Here's how the part is built. I have some questions about the finished solid (model axes, mm). Coordinates: 2 decimals unless noted, no trailing zeros. Write each loop counter-clockwise with the first axis right and the second up, starting at its lowest first coordinate (ties: lowest second). Pieces come first, ordered by that corner, then holes.
Item 1: We'd pull the mould along Z, two halves only. Please class faces 1 (the face through (0, 1, 400)), 2 (the face through (-0.705, 3.479, 88.173)), 3 (the face through (1.4, 1.958, 61.4)), 4 (the face through (0, 4.958, 197)): +Z half, -Z half, draft (parallel to the pull), parting line (faces both ways), or undercut.
Item 2: I'm going to push flat-ended pins straight in: pin 1 Ø1 at (x, z) = (-2.5, 260.5) entering from +Y; pin 2 Ø3 at (y, z) = (2.5, 318.5) entering from -X; pin 3 Ø3 at (x, z) = (0, 135) entering from +Y. Where does each tip first touch, or does it pass through?
Item 3: If we section it at A-A (y = 3.5): Count the separate pieces of the cut face and the enclosed holes in it, then the cut area to 3 significant figures.
Item 4: If I drill on line 1 (X direction, y = 2, z = 21); line 2 (X direction, y = 3.3, z = 235); line 3 (X direction, y = 2.5, z = 159), over which ranges is the centre line in solid material (lowest first)?
Item 5: If we section it at B-B (z = 48.5): Please give me the cut outline in (x, y).
from build123d import *

# Parameters (mm, degrees)
EXTRUDE_1_DEPTH              = 400
HOLE_WIZARD_M3_1_D           = 3.4
HOLE_WIZARD_M3_1_CBORE_D     = 6.5
HOLE_WIZARD_M3_1_CBORE_DEPTH = 3


with BuildPart() as part:
    # 草图1 → 凸台-拉伸1 (new body)
    with BuildSketch(Plane(origin=(0, 0, 0), x_dir=(-1, 0, 0), z_dir=(0, 0, -1))):
        Polygon((-4, 4.958168347), (-5.3, 1.958168347), (-3, 0.958168347), (-6, -0.041831653), (-6, -2.974901007), (6, -2.974901007), (6, -0.041831653), (3, 0.958168347), (5.3, 1.958168347), (4, 4.958168347), align=None)
    extrude(amount=-EXTRUDE_1_DEPTH)

    # M3 六角头机械螺钉的柱形沉头孔1 (through all)
    with Locations(Plane(origin=(0, 4.958168347, 0), x_dir=(1, 0, 0), z_dir=(0, 1, 0))):
        with Locations((0, -385), (0, -360), (0, -335), (0, -310), (0, -285), (0, -260), (0, -235), (0, -210), (0, -185), (0, -160), (0, -135), (0, -110), (0, -85), (0, -60), (0, -10), (0, -35)):
            CounterBoreHole(HOLE_WIZARD_M3_1_D / 2, HOLE_WIZARD_M3_1_CBORE_D / 2, HOLE_WIZARD_M3_1_CBORE_DEPTH)


solid = part.part
Answer list:
1. face 1: +Z half
1. face 2: undercut
1. face 3: undercut
1. face 4: draft
2. pin 1: stops at y = 1.96
2. pin 2: stops at x = -5.3
2. pin 3: passes through
3. separate pieces: 1
3. enclosed holes: 16
3. area: 3,170 mm2
4. line 1: x = -5.28 to 5.28
4. line 2: x = -4.72 to -3.25, 3.25 to 4.72
4. line 3: x = -5.07 to -3.09, 3.09 to 5.07
5. outline: (-6, -2.97) - (6, -2.97) - (6, -0.04) - (3, 0.96) - (5.3, 1.96) - (4, 4.96) - (-4, 4.96) - (-5.3, 1.96) - (-3, 0.96) - (-6, -0.04) - close
